Job drawing, mm, ordinate dimensions from the low corner. One solid piece. A direction names the side the tool comes from. Give positions to 0.01 mm unless a question says otherwise; leave off trailing zeros. Order: outer loops, then holes, each group sorted by start corner. A loop starts at its lowest first (then second) coordinate and runs counter-clockwise, first axis right, second up.
Item 1: Flat gauge pins, fed straight in: P1, Ø4, axis at x = 20, z = 6, coming from the +Y side; P2, Ø1.5, axis at x = 19.5, y = 20.5, coming from the -Z side; P3, Ø12, axis at x = 30.5, y = 10.5, coming from the -Z side. Where does each tip first touch, or does it go through?
Item 2: Band-saw the part on C-C on z = 13. Give the cut face in (x, y) (1 decimal).
Item 3: Wall check: L1, parallel to X at y = 27, z = 20; L2, parallel to X at y = 3, z = 13 (1 decimal); L3, parallel to Y at x = 17, z = 10.5. Give the ranges that are in metal, low to high.
Item 4: Two-plate mould, pull along X, no slides. Class the marked faces 3, 4 and 5: released by +X, released by -X, zero draft, split by the parting line, or undercut.
Item 5: Band-saw the part on D-D on y = 36. Give the cut face in (x, z).
Item 6: Which spindle directions (+Z, -Z, +X, -X, +Y, -Y) get a long thin tool onto all of the face, cutting with end or side? Do the marked faces 1 and 2. Say none if no direction does.
Item 7: Band-saw the part on A-A on x = 20. Give the cut face in (y, z), plus the area to 3 significant figures.
Item 8: Band-saw the part on B-B on z = 19. Give the cut face in (x, y) (1 decimal), plus the area to 3 significant figures.
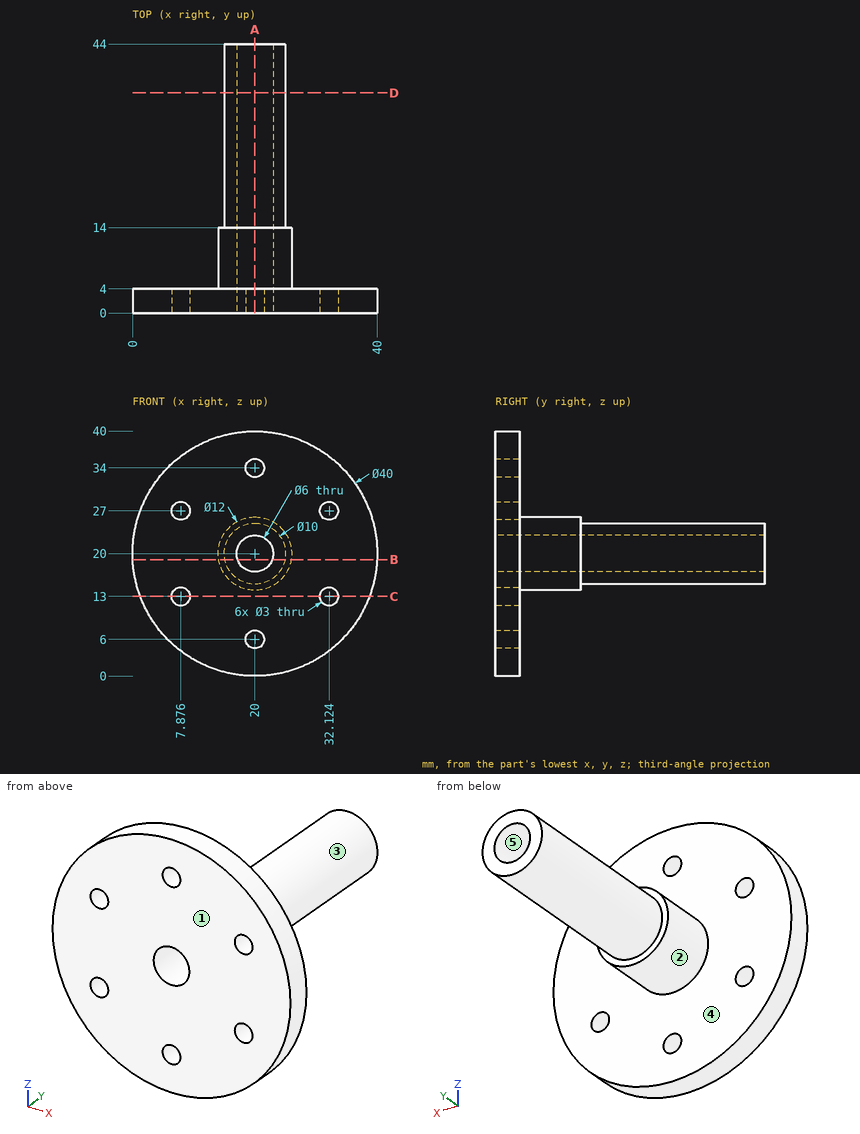
The answers:
1. P1: stops at y = 4
1. P2: stops at z = 15
1. P3: stops at z = 16.03
2. outline: (1.3, 0) - (6.4, 0) - (6.4, 4) - (1.3, 4) - close; (9.4, 0) - (30.6, 0) - (30.6, 4) - (9.4, 4) - close; (33.6, 0) - (38.7, 0) - (38.7, 4) - (33.6, 4) - close
3. L1: x = 15 to 17, 23 to 25
3. L2: x = 1.3 to 6.4, 9.4 to 30.6, 33.6 to 38.7
3. L3: y = 0 to 4
4. face 3: split by the parting line
4. face 4: zero draft
4. face 5: undercut
5. outline: circle Ø10 at (20, 20); hole circle Ø6 at (20, 20)
6. face 1: +Z, -Z, +X, -X, -Y
6. face 2: +Y
7. outline: (0, 0) - (4, 0) - (4, 4.5) - (0, 4.5) - close; (0, 7.5) - (4, 7.5) - (4, 14) - (14, 14) - (14, 15) - (44, 15) - (44, 17) - (0, 17) - close; (0, 23) - (44, 23) - (44, 25) - (14, 25) - (14, 26) - (4, 26) - (4, 32.5) - (0, 32.5) - close; (0, 35.5) - (4, 35.5) - (4, 40) - (0, 40) - close
7. area: 292 mm2
8. outline: (0, 0) - (17.2, 0) - (17.2, 44) - (15.1, 44) - (15.1, 14) - (14.1, 14) - (14.1, 4) - (0, 4) - close; (22.8, 0) - (40, 0) - (40, 4) - (25.9, 4) - (25.9, 14) - (24.9, 14) - (24.9, 44) - (22.8, 44) - close
8. area: 323 mm2
